For this review, take the finished solid that the model builds, in its own axes (mm). A direction names the side the tool comes from. Coordinates: 2 decimals unless noted, no trailing zeros. Write each loop counter-clockwise with the first axis right and the second up, starting at its lowest first coordinate (ties: lowest second). Pieces come first, ordered by that corner, then holes. Notation, with made-up numbers: (-38, 1.25) - (-30, 1.25) arc R34 cw to (-30, 35.25) - close; hole circle Ø11 at (-35, 21). An arc over 180 degrees is marked (long way). Write each question's results on one line, items separated by ' | '.
from build123d import *

# Parameters (mm, degrees)
SKIZZE1_R                        = 34
AUFSATZ_LINEAR_AUSTRAGEN1_DEPTH  = 10
SKIZZE3_R                        = 42.5
AUFSATZ_LINEAR_AUSTRAGEN2_DEPTH  = 5
F_15_0_15_DURCHMESSER_BOHRUNG1_D = 15
F_5_5_5_5_DURCHMESSER_BOHRUNG1_D = 5.5


with BuildPart() as part:
    # Skizze1 → Aufsatz-Linear austragen1 (new body)
    with BuildSketch(Plane.XY):
        Circle(SKIZZE1_R)
    extrude(amount=AUFSATZ_LINEAR_AUSTRAGEN1_DEPTH)

    # Skizze3 → Aufsatz-Linear austragen2 (add)
    with BuildSketch(Plane(origin=(0, 0, 0), x_dir=(-1, 0, 0), z_dir=(0, 0, -1))):
        Circle(SKIZZE3_R)
    extrude(amount=AUFSATZ_LINEAR_AUSTRAGEN2_DEPTH)

    # Ø15.0 (15) Durchmesser Bohrung1 (through all)
    with Locations(Plane(origin=(0, 0, -5), x_dir=(-1, 0, 0), z_dir=(0, 0, -1))):
        with Locations((0, 0)):
            Hole(F_15_0_15_DURCHMESSER_BOHRUNG1_D / 2)

    # Ø5.5 (5.5) Durchmesser Bohrung1 (through all)
    with Locations(Plane(origin=(0, 0, -5), x_dir=(-1, 0, 0), z_dir=(0, 0, -1))):
        with Locations((18, 0), (-18, 0)):
            Hole(F_5_5_5_5_DURCHMESSER_BOHRUNG1_D / 2)


solid = part.part
Q1. Take a section at C-C on z = 4.75. State the section outline as (x, y) points.
Results found:
outline: circle Ø68 at (0, 0); hole circle Ø5.5 at (-18, 0); hole circle Ø15 at (0, 0); hole circle Ø5.5 at (18, 0)
Q2. For faces 4 (the face through (-7.493, 0.33, 2.605)), 5 (the face through (19, 29, 0)), list the 3-axis set-ups (+Z, -Z, +X, -X, +Y, -Y) from which the entire face can be reached by the end or side of a thin tool; tool diameter is ignored.
Results found:
face 4: +Z, -Z | face 5: +Z
Q3. Take a section at A-A on y = 0. State the section outline as (x, z) points.
Results found:
outline: (-42.5, -5) - (-20.75, -5) - (-20.75, 10) - (-34, 10) - (-34, 0) - (-42.5, 0) - close; (-15.25, -5) - (-7.5, -5) - (-7.5, 10) - (-15.25, 10) - close; (7.5, -5) - (15.25, -5) - (15.25, 10) - (7.5, 10) - close; (20.75, -5) - (42.5, -5) - (42.5, 0) - (34, 0) - (34, 10) - (20.75, 10) - close
Q4. For pin 1 (5 mm diameter, centred on y = -32, z = -1.5, fed in from -X); pin 2 (4 mm diameter, centred on x = 18, z = -0.5, fed in from -Y); pin 3 (2 mm diameter, centred on y = 21, z = -0.5, fed in from +X), all flat-tipped, find the tip position at first contact; note any pin that passes through.
Results found:
pin 1: x = -30.59 | pin 2: y = -39.37 | pin 3: x = 37.5
Q5. Wall thickness on line 1 along Y through (x, z) = (0, 2.5); line 2 along Y through (x, z) = (25.5, -4); line 3 along Y through (x, z) = (-18, 1.5): over which ranges is each line inside the solid? List them lowest first. Write a range as from..to.
Results found:
line 1: -34..-7.5, 7.5..34 | line 2: -34..34 | line 3: -28.84..-2.75, 2.75..28.84
Q6. Mouldability with a two-part tool opening along Y and no side actions: class faces 1 (the face through (1, -9, -5)), 2 (the face through (-20.747, 0.121, 2.605)), 3 (the face through (18.28, 28.67, 4.93)) as pulls with the +Y half, pulls with the -Y half, needs draft (parallel to the pull), parting line crosses it, or undercut.
Results found:
face 1: needs draft | face 2: undercut | face 3: parting line crosses it
Q7. Take a section at B-B on x = 0. State the section outline as (y, z) points.
Results found:
outline: (-42.5, -5) - (-7.5, -5) - (-7.5, 10) - (-34, 10) - (-34, 0) - (-42.5, 0) - close; (7.5, -5) - (42.5, -5) - (42.5, 0) - (34, 0) - (34, 10) - (7.5, 10) - close
Q8. Take a section at D-D on y = -12.5. State the section outline as (x, z) points, plus the area to 3 significant figures.
Results found:
outline: (-40.62, -5) - (40.62, -5) - (40.62, 0) - (31.62, 0) - (31.62, 10) - (-31.62, 10) - (-31.62, 0) - (-40.62, 0) - close | area: 1,040 mm2
